The figure shows three views and two pictorial views of one solid part (mm, origin at its lowest corner). Answer the questions. A direction names the side the tool comes from. Give positions to 0.01 mm unless a question says otherwise; leave off trailing zeros. Order: outer loops, then holes, each group sorted by start corner. A loop starts at its lowest first (then second) coordinate and runs counter-clockwise, first axis right, second up. Notation, with made-up numbers: (46, 28.25) - (71, 28.25) arc R8 ccw to (71, 41.25) - close; hole circle Ø4 at (-12, 22.5). An arc over 180 degrees is marked (long way). Answer as a JSON object with one key per item and string values. Group by question number.
Q1. Given pin 1 (1.7 mm diameter, centred on x = 20, z = 1, fed in from +Y); pin 2 (1.5 mm diameter, centred on x = 14.5, z = 5, fed in from +Y); pin 3 (1 mm diameter, centred on y = 27, z = 12, fed in from -X); pin 4 (9.5 mm diameter, centred on x = 16.5, y = 15.5, fed in from +Z), each flat-ended and moving along its own axis, determine where each tip first touches the part or whether it passes through.
Q2. A cutting plane is placed at B-B, the plane y = 25. Give the vertices of the cut face in (x, z).
Q3. Consider line 1 (Y direction, x = 3, z = 7.25); line 2 (Z direction, x = 21, y = 3.5); line 3 (Y direction, x = 29, z = 4.5). Determine where each line is inside the solid, lowest interval first.
Q4. A cutting plane is placed at A-A, the plane z = 7.25. Give the vertices of the cut face in (x, y), and give its area (3 significant figures).
Q5. A cutting plane is placed at C-C, the plane x = 21. Give the vertices of the cut face in (y, z).
Q6. For the marked faces 1, 2 and 3, determine the directions among +Z, -Z, +X, -X, +Y, -Y from which every point of the face is accessible in a straight line to the end or side of a thin tool.
Q7. A cutting plane is placed at D-D, the plane y = 5. Give the vertices of the cut face in (x, z).
Q8. The mould has two halves that part along Y. Classify the marked faces 4, 5, 6 and 7: released by +Y, released by -Y, zero draft, split by the parting line, or undercut.
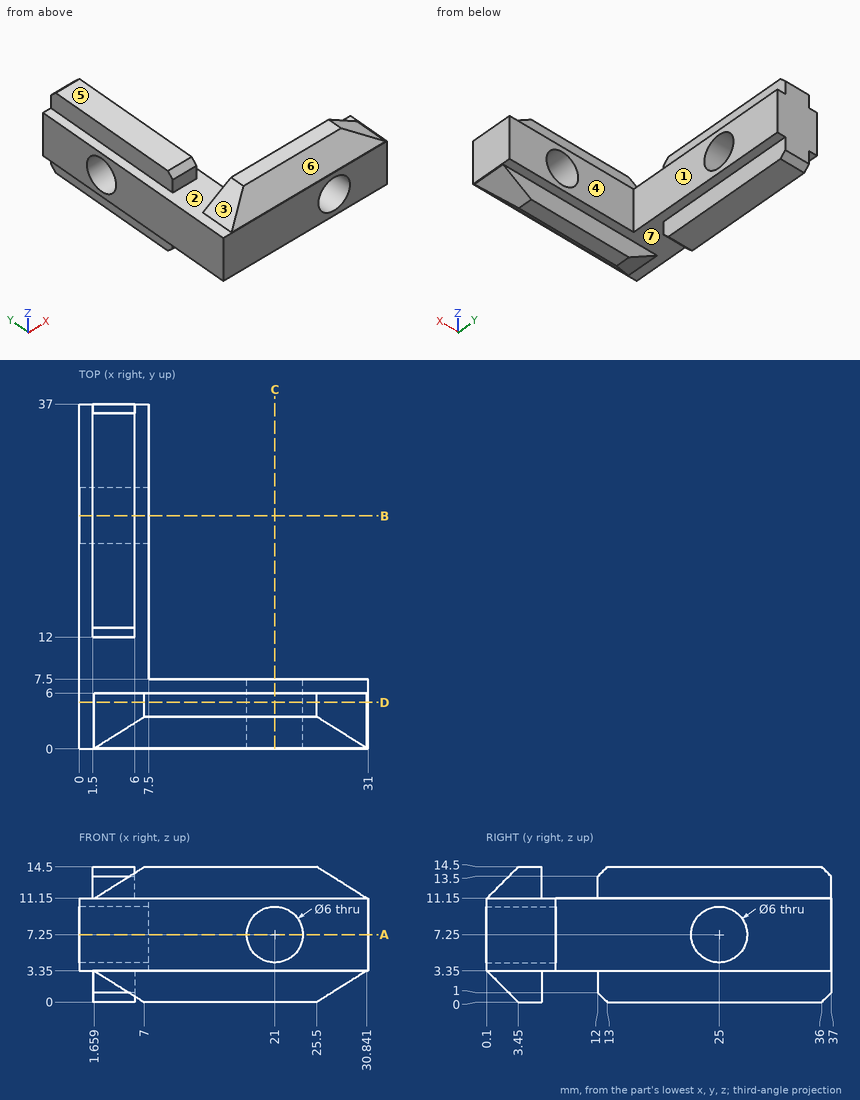
Reply:
{
 "1": {"pin 1": "stops at y = 6", "pin 2": "stops at y = 7.5", "pin 3": "stops at x = 1.5", "pin 4": "passes through"},
 "2": {"outline": "(0, 3.35) - (1.5, 3.35) - (1.5, 0) - (6, 0) - (6, 3.35) - (7.5, 3.35) - (7.5, 4.25) - (0, 4.25) - close; (0, 10.25) - (7.5, 10.25) - (7.5, 11.15) - (6, 11.15) - (6, 14.5) - (1.5, 14.5) - (1.5, 11.15) - (0, 11.15) - close"},
 "3": {"line 1": "y = 0 to 22, 28 to 37", "line 2": "z = 0 to 4.25, 10.25 to 14.5", "line 3": "y = 0 to 7.5"},
 "4": {"outline": "(0, 0) - (18, 0) - (18, 7.5) - (7.5, 7.5) - (7.5, 22) - (0, 22) - close; (0, 28) - (7.5, 28) - (7.5, 37) - (0, 37) - close; (24, 0) - (31, 0) - (31, 7.5) - (24, 7.5) - close", "area": "364 mm^2"},
 "5": {"outline": "(0, 3.35) - (0.1, 3.35) - (3.45, 0) - (6, 0) - (6, 3.35) - (7.5, 3.35) - (7.5, 4.25) - (0, 4.25) - close; (0, 10.25) - (7.5, 10.25) - (7.5, 11.15) - (6, 11.15) - (6, 14.5) - (3.45, 14.5) - (0.1, 11.15) - (0, 11.15) - close"},
 "6": {"face 1": "+Z, -Z, +X, +Y", "face 2": "+Z", "face 3": "+Z, -X, -Y"},
 "7": {"outline": "(0, 3.35) - (1.66, 3.35) - (7, 0) - (25.5, 0) - (30.84, 3.35) - (31, 3.35) - (31, 11.15) - (30.84, 11.15) - (25.5, 14.5) - (7, 14.5) - (1.66, 11.15) - (0, 11.15) - close; hole circle Ø6 at (21, 7.25)"},
 "8": {"face 4": "released by +Y", "face 5": "zero draft", "face 6": "released by -Y", "face 7": "undercut"}
}
